Geometry: final body of the model. Coordinates: model frame, mm. Round coordinates to 2 decimals unless told otherwise and drop trailing zeros. Write each loop counter-clockwise with the first axis right and the second up, starting at its lowest first coordinate (ties: lowest second). Pieces come first, ordered by that corner, then holes. Notation, with made-up numbers: (81, 46) - (101, 46) arc R19 cw to (101, 57) - close; hole circle Ø11 at (45, 13.25). An arc over 180 degrees is marked (long way). Use a Markdown table: item, result. Add a question column.
```python
from build123d import *

# Parameters (mm, degrees)
SKETCH1_W           = 130
SKETCH1_H           = 50
SKETCH1_R           = 2.5
SKETCH1_R_2         = 3.5
SKETCH1_W_2         = 110
SKETCH1_H_2         = 10
BOSS_EXTRUDE2_DEPTH = 10
FILLET1_R           = 10


with BuildPart() as part:
    # Sketch1 → Boss-Extrude2 (new body)
    with BuildSketch(Plane.XY):
        with Locations((65, 25)):
            Rectangle(SKETCH1_W, SKETCH1_H)
        with Locations((36.53, 41.03)):
            Circle(SKETCH1_R, mode=Mode.SUBTRACT)
        with Locations((93.47, 41.03)):
            Circle(SKETCH1_R, mode=Mode.SUBTRACT)
        with Locations((65, 7)):
            Circle(SKETCH1_R_2, mode=Mode.SUBTRACT)
        with Locations((65, 30)):
            Rectangle(SKETCH1_W_2, SKETCH1_H_2, mode=Mode.SUBTRACT)
    extrude(amount=BOSS_EXTRUDE2_DEPTH)

    # Fillet1
    fillet1_edges = [part.edges().sort_by_distance(p)[0] for p in [
        (0, 50, 5),
        (130, 50, 5),
        (130, 0, 5),
        (0, 0, 5),
    ]]
    fillet(fillet1_edges, radius=FILLET1_R)


solid = part.part
```
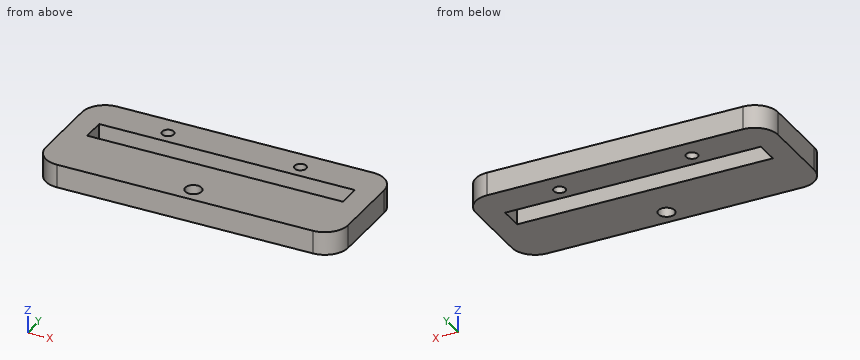
1) Section C-C, the plane y = 32. Return the cut outline in (x, z).
2) Material intervals for L1, parallel to Y at x = 36.53, z = 3.25; L2, parallel to Y at x = 65, z = 2.5; L3, parallel to Y at x = 46, z = 5.5, sorted ascending. Write a range as from..to.
3) Section D-D, the plane z = 3.5. Return the cut outline in (x, y).
4) Section A-A, the plane x = 36.53. Return the cut outline in (y, z).
5) Section B-B, the plane x = 13. Return the cut outline in (y, z).
Output values:
| question | item | result |
|---|---|---|
| 1 | outline | (0, 0) - (10, 0) - (10, 10) - (0, 10) - close; (120, 0) - (130, 0) - (130, 10) - (120, 10) - close |
| 2 | L1 | y = 0..25, 35..38.53, 43.53..50 |
| 2 | L2 | y = 0..3.5, 10.5..25, 35..50 |
| 2 | L3 | y = 0..25, 35..50 |
| 3 | outline | (0, 10) arc R10 ccw to (10, 0) - (120, 0) arc R10 ccw to (130, 10) - (130, 40) arc R10 ccw to (120, 50) - (10, 50) arc R10 ccw to (0, 40) - close; hole (10, 25) - (120, 25) - (120, 35) - (10, 35) - close; hole circle Ø5 at (36.53, 41.03); hole circle Ø7 at (65, 7); hole circle Ø5 at (93.47, 41.03) |
| 4 | outline | (0, 0) - (25, 0) - (25, 10) - (0, 10) - close; (35, 0) - (38.53, 0) - (38.53, 10) - (35, 10) - close; (43.53, 0) - (50, 0) - (50, 10) - (43.53, 10) - close |
| 5 | outline | (0, 0) - (25, 0) - (25, 10) - (0, 10) - close; (35, 0) - (50, 0) - (50, 10) - (35, 10) - close |
